```python
from build123d import *

# Parameters (mm, degrees)
SKETCH_1_W          = 62
SKETCH_1_H          = 56
EXTRUDE_1_DEPTH     = 2
SKETCH_2_R          = 1.6
CUT_EXTRUDE_1_DEPTH = 2
SKETCH_3_R          = 1
CUT_EXTRUDE_2_DEPTH = 84.570329663


with BuildPart() as part:
    # Эскиз1 → Бобышка-Вытянуть1 (new body)
    with BuildSketch(Plane(origin=(0, 0, 0), x_dir=(1, 0, 0), z_dir=(0, 1, 0))):
        with Locations((31, -28)):
            Rectangle(SKETCH_1_W, SKETCH_1_H)
    extrude(amount=EXTRUDE_1_DEPTH)

    # Эскиз2 → Вырез-Вытянуть1 (cut)
    with BuildSketch(Plane(origin=(0, 2, 0), x_dir=(1, 0, 0), z_dir=(0, 1, 0))):
        with Locations(Location((6.7, -7.2, 0), (0, 0, 270))):
            Circle(SKETCH_2_R)
        with Locations(Location((6.7, -51.8, 0), (0, 0, 270))):
            Circle(SKETCH_2_R)
        with Locations(Location((57.4, -51.8, 0), (0, 0, 270))):
            Circle(SKETCH_2_R)
        with Locations(Location((57.4, -8.4, 0), (0, 0, 270))):
            Circle(SKETCH_2_R)
    extrude(amount=-CUT_EXTRUDE_1_DEPTH, mode=Mode.SUBTRACT)

    # Эскиз3 → Вырез-Вытянуть2 (cut, through all)
    with BuildSketch(Plane(origin=(0, 2, 0), x_dir=(1, 0, 0), z_dir=(0, 1, 0))):
        with Locations(Location((5.5, -32.8, 0), (0, 0, 270))):
            Circle(SKETCH_3_R)
        with Locations(Location((5.5, -42, 0), (0, 0, 270))):
            Circle(SKETCH_3_R)
        with Locations(Location((26.2, -51.2, 0), (0, 0, 270))):
            Circle(SKETCH_3_R)
        with Locations(Location((35.6, -51.2, 0), (0, 0, 270))):
            Circle(SKETCH_3_R)
        with Locations(Location((44.9, -51.2, 0), (0, 0, 270))):
            Circle(SKETCH_3_R)
    extrude(amount=-CUT_EXTRUDE_2_DEPTH, mode=Mode.SUBTRACT)


solid = part.part
```
Design review of the part built by this model. Coordinates are the model's own, in mm. Coordinates: 2 decimals unless noted, no trailing zeros. Write each loop counter-clockwise with the first axis right and the second up, starting at its lowest first coordinate (ties: lowest second). Pieces come first, ordered by that corner, then holes. Notation, with made-up numbers: M -13.5,76.25 L 10.5,76.25 A20 ccw 10.5,90.25 Z; hole C -37.5,76 d5. An arc over 180 degrees is marked long. Answer as a JSON object with one key per item and string values.
Item 1: Add section A-A, the plane x = 35.6. Give the boundary of the cut face in (y, z), and give its area (3 significant figures).
Outcome:
{"outline": "M 0,0 L 2,0 L 2,50.2 L 0,50.2 Z; M 0,52.2 L 2,52.2 L 2,56 L 0,56 Z", "area": "108 mm²"}
Item 2: Draft analysis for pull direction X (two halves, no side actions). For faces 1 (the flat face through (0, 1, 28)), 2 (the cylindrical face through (44.3, 1, 50.4)), 3 (the flat face through (31, 2, 28)), state which applies: pulls with the +X half, pulls with the -X half, needs draft (parallel to the pull), parting line crosses it, or undercut.
Outcome:
{"face 1": "pulls with the -X half", "face 2": "undercut", "face 3": "needs draft"}
Item 3: Add section C-C, the plane x = 57.4. Give the boundary of the cut face in (y, z).
Outcome:
{"outline": "M 0,0 L 2,0 L 2,6.8 L 0,6.8 Z; M 0,10 L 2,10 L 2,50.2 L 0,50.2 Z; M 0,53.4 L 2,53.4 L 2,56 L 0,56 Z"}
Item 4: Add section B-B, the plane z = 42. Give the boundary of the cut face in (x, y), and give its area (3 significant figures).
Outcome:
{"outline": "M 0,0 L 4.5,0 L 4.5,2 L 0,2 Z; M 6.5,0 L 62,0 L 62,2 L 6.5,2 Z", "area": "120 mm²"}
Item 5: Wall thickness on probe 1 along Z at (x, y) = (57.5, 0.8); probe 2 along X at (y, z) = (0.75, 42); probe 3 along X at (y, z) = (1.6, 8.4): over which ranges is each line inside the solid? List them lowest first.
Outcome:
{"probe 1": "0 to 6.8, 10 to 50.2, 53.4 to 56", "probe 2": "0 to 4.5, 6.5 to 62", "probe 3": "0 to 5.64, 7.76 to 55.8, 59 to 62"}
Item 6: Add section D-D, the plane z = 51.2. Give the boundary of the cut face in (x, y), and give its area (3 significant figures).
Outcome:
{"outline": "M 0,0 L 5.22,0 L 5.22,2 L 0,2 Z; M 8.18,0 L 25.2,0 L 25.2,2 L 8.18,2 Z; M 27.2,0 L 34.6,0 L 34.6,2 L 27.2,2 Z; M 36.6,0 L 43.9,0 L 43.9,2 L 36.6,2 Z; M 45.9,0 L 55.92,0 L 55.92,2 L 45.9,2 Z; M 58.88,0 L 62,0 L 62,2 L 58.88,2 Z", "area": "100 mm²"}
Item 7: Insertion check: pin 1 Ø1.6 at (x, z) = (5.5, 42) entering from +Y. The pin has a flat end and moves straight along its axis. Give the tip position at first contact, or say it passes through.
Outcome:
{"pin 1": "through"}
